```python
from build123d import *

# Parameters (mm, degrees)
SKETCH1_W                                 = 16
SKETCH1_H                                 = 16
BASE_DEPTH                                = 50
SKETCH2_W                                 = 2
SKETCH2_H                                 = 16
RODSLOT_DEPTH                             = 54.103672189
F_5_1_5_1_FREE_HOLE_FOR_SCREW_D           = 5.1
F_5_1_5_1_FREE_HOLE_FOR_SCREW_DEPTH       = 7.5
F_5_1_5_1_FREE_HOLE_FOR_SCREW_CSINK_D     = 6.1
F_5_1_5_1_FREE_HOLE_FOR_SCREW_CSINK_ANGLE = 90
F_5_1_5_1_FREE_HOLE_FOR_SCREW_TIP         = 1.056244584
M5X0_8_TAPPED_HOLE_FOR_ROD_SCREW_D        = 4.2
M5X0_8_TAPPED_HOLE_FOR_ROD_SCREW_DEPTH    = 7.6381927
M5X0_8_TAPPED_HOLE_FOR_ROD_SCREW_TIP      = 1.2618073
F_3_1_3_1_SCREW_HOLES_D                   = 3.1
F_10_2_10_2_ROD_HOLE_D                    = 10.2


with BuildPart() as part:
    # Sketch1 → Base (new body)
    with BuildSketch(Plane.XY):
        Rectangle(SKETCH1_W, SKETCH1_H)
    extrude(amount=BASE_DEPTH)

    # Sketch2 → RodSlot (cut, through all)
    with BuildSketch(Plane(origin=(0, 8, 0), x_dir=(1, 0, 0), z_dir=(0, 1, 0))):
        with Locations((0, -42)):
            Rectangle(SKETCH2_W, SKETCH2_H)
    extrude(amount=-RODSLOT_DEPTH, mode=Mode.SUBTRACT)

    # Ø5.1 (5.1) free hole for screw
    with Locations(Plane(origin=(8, 0, 0), x_dir=(0, 0, -1), z_dir=(1, 0, 0))):
        with Locations((-45, 0)):
            CounterSinkHole(F_5_1_5_1_FREE_HOLE_FOR_SCREW_D / 2, F_5_1_5_1_FREE_HOLE_FOR_SCREW_CSINK_D / 2, depth=F_5_1_5_1_FREE_HOLE_FOR_SCREW_DEPTH, counter_sink_angle=F_5_1_5_1_FREE_HOLE_FOR_SCREW_CSINK_ANGLE)
            with Locations((0, 0, -(F_5_1_5_1_FREE_HOLE_FOR_SCREW_DEPTH + F_5_1_5_1_FREE_HOLE_FOR_SCREW_TIP / 2))):  # 135° drill point
                Cone(0, F_5_1_5_1_FREE_HOLE_FOR_SCREW_D / 2, F_5_1_5_1_FREE_HOLE_FOR_SCREW_TIP, mode=Mode.SUBTRACT)

    # M5x0.8 Tapped Hole for rod screw
    with Locations(Plane.ZY.offset(8)):
        with Locations((45, 0)):
            Hole(M5X0_8_TAPPED_HOLE_FOR_ROD_SCREW_D / 2, depth=M5X0_8_TAPPED_HOLE_FOR_ROD_SCREW_DEPTH)
            with Locations((0, 0, -(M5X0_8_TAPPED_HOLE_FOR_ROD_SCREW_DEPTH + M5X0_8_TAPPED_HOLE_FOR_ROD_SCREW_TIP / 2))):  # 118° drill point
                Cone(0, M5X0_8_TAPPED_HOLE_FOR_ROD_SCREW_D / 2, M5X0_8_TAPPED_HOLE_FOR_ROD_SCREW_TIP, mode=Mode.SUBTRACT)

    # Ø3.1 (3.1) screw holes (through all)
    with Locations(Plane(origin=(0, -8, 0), x_dir=(-1, 0, 0), z_dir=(0, -1, 0))):
        with Locations((3, -5), (-3, -11)):
            Hole(F_3_1_3_1_SCREW_HOLES_D / 2)

    # Ø10.2 (10.2) Rod Hole (through all)
    with Locations(Plane(origin=(0, 8, 0), x_dir=(1, 0, 0), z_dir=(0, 1, 0))):
        with Locations((0, -30)):
            Hole(F_10_2_10_2_ROD_HOLE_D / 2)


solid = part.part
```
Geometry check sheet. Reference: the model listing, model coordinates, mm. A direction names the side the tool comes from. Coordinates: 2 decimals unless noted, no trailing zeros. Order: outer loops, then holes, each group sorted by start corner. A loop starts at its lowest first (then second) coordinate and runs counter-clockwise, first axis right, second up.
Item 1: Scan lines: line 1 along Y through (x, z) = (2.25, 45); line 2 along Z through (x, y) = (-3, 2.75); line 3 along Z through (x, y) = (-3, -1.75). Record each from-to range of solid material in increasing order.
Item 2: Mould release check, pull along X, two halves, no side actions. Record for faces 1 (the flat face through (0, 0, 0)), 2 (the cylindrical face through (-4.55, 0.11, 4.93)), 3 (the flat face through (8, 0, 25)): released by +X, released by -X, zero draft, split by the parting line, or undercut.
Item 3: Tool access check on faces 4 (the cylindrical face through (-4.45, -0.8, 43.06)), 5 (the cylindrical face through (4.204, 0.112, 42.452)), 6 (the flat face through (1, 0, 41)). Record the directions out of +Z, -Z, +X, -X, +Y, -Y that give a thin tool (end or side, any length) a straight path to the whole face; none if there is none.
Item 4: Depth check by flat-ended pin: pin 1 (5.5 mm diameter, centred on y = 0, z = 45, fed in from +X). Enter the tip coordinate at first touch or a pass-through.
Item 5: Section check D-D (y = 3.5). Enter the section's corners in (x, z).
Item 6: Section check A-A (y = 0). Enter the section's corners in (x, z), plus the area to 3 significant figures.
Item 7: Section check C-C (z = 5). Enter the section's corners in (x, y), plus the area to 3 significant figures.
Item 8: Section check B-B (x = -2.25). Enter the section's corners in (y, z), plus the area to 3 significant figures.
Check sheet entries:
1. line 1: y = -8 to -2.55, 2.55 to 8
1. line 2: z = 0 to 3.45, 6.55 to 25.88, 34.12 to 50
1. line 3: z = 0 to 3.45, 6.55 to 25.88, 34.12 to 43.84, 46.16 to 50
2. face 1: zero draft
2. face 2: undercut
2. face 3: released by +X
3. face 4: +X, -X
3. face 5: +X
3. face 6: +Z, +Y, -Y
4. pin 1: stops at x = 7.7
5. outline: (-8, 0) - (8, 0) - (8, 50) - (1, 50) - (1, 35) arc R5.1 cw (long way) to (-1, 35) - (-1, 50) - (-8, 50) - close; hole circle Ø3.1 at (-3, 5); hole circle Ø3.1 at (3, 11)
6. outline: (-8, 0) - (8, 0) - (8, 41.95) - (7.5, 42.45) - (1, 42.45) - (1, 35) arc R5.1 cw (long way) to (-1, 35) - (-1, 42.9) - (-8, 42.9) - close; (-8, 47.1) - (-1, 47.1) - (-1, 50) - (-8, 50) - close; (1, 47.55) - (7.5, 47.55) - (8, 48.05) - (8, 50) - (1, 50) - close; hole circle Ø3.1 at (-3, 5); hole circle Ø3.1 at (3, 11)
6. area: 608 mm2
7. outline: (-8, -8) - (-4.55, -8) - (-4.55, 8) - (-8, 8) - close; (-1.45, -8) - (8, -8) - (8, 8) - (-1.45, 8) - close
7. area: 206 mm2
8. outline: (-8, 0) - (8, 0) - (8, 3.64) - (-8, 3.64) - close; (-8, 6.36) - (8, 6.36) - (8, 25.42) - (-8, 25.42) - close; (-8, 34.58) - (8, 34.58) - (8, 50) - (-8, 50) - close; hole circle Ø4.2 at (0, 45)
8. area: 596 mm2
